Source: CAD feature listing. Evaluate the final solid. Frame: model axes, mm. A direction names the side the tool comes from. Coordinates: 2 decimals unless noted, no trailing zeros. Order: outer loops, then holes, each group sorted by start corner. A loop starts at its lowest first (then second) coordinate and runs counter-clockwise, first axis right, second up.
Autodesk Inventor part; units mm, degrees
ref_plane "YZ Plane" through (0, 0, 0) normal (1, 0, 0) x (0, 1, 0)
ref_plane "XZ Plane" through (0, 0, 0) normal (0, 1, 0) x (-1, 0, 0)
ref_plane "XY Plane" through (0, 0, 0) normal (0, 0, 1) x (1, 0, 0)
sketch "Sketch1" plane through (0, 0, 0) normal (0, 0, 1) x (1, 0, 0)
  line L0 (-16.8009, 21.2415) -> (21.2415, -16.8009)
  line L1 (21.2415, -16.8009) -> (16.8009, -21.2415)
  line L2 (16.8009, -21.2415) -> (-21.2415, 16.8009)
  line L3 (-21.2415, 16.8009) -> (-16.8009, 21.2415)
  line L4 (-16.8009, 21.2415) -> (16.8009, -21.2415) construction
  line L5 (21.2415, -16.8009) -> (-21.2415, 16.8009) construction
  line L6 (-16.8009, 21.2415) -> (36.9991, 21.2415) construction
  line L7 (-21.2415, 16.8009) -> (-24, 16.8009)
  line L8 (16.8009, -21.2415) -> (16.8009, -24)
  line L9 (16.8009, -24) -> (-24, 16.8009)
  line L10 (-16.8009, 21.2415) -> (-16.8009, 24)
  line L11 (21.2415, -16.8009) -> (24, -16.8009)
  line L12 (24, -16.8009) -> (-16.8009, 24)
  line L13 (-24, 16.8009) -> (-24, 12.6863)
  line L14 (16.8009, -24) -> (12.6863, -24)
  line L15 (-24, 12.6863) -> (12.6863, -24)
  line L16 (-24, 16.8009) -> (-11.8721, 28.9288) construction
  line L17 (-24, 16.8009) -> (-6.8486, 16.8009) construction
  point P0 (0, 0)
  dimension "d0" = 53.8
  dimension "d1" = 45
  dimension "d2" = 6.28
  dimension "d5" = 8
  dimension "d72" = 24
  dimension "d73" = 45
extrude "Extrusion1" add sketch "Sketch1" along normal blind 30
ref_plane "Work Plane1" through (16.9, -16.9, -8) normal (-0.7071, -0.7071, 0) x (0, 0, 1)
sketch "Sketch7" plane through (0, 0, 30) normal (0, 0, 1) x (1, 0, 0)
  line L0 (21.2415, -16.8009) -> (24, -16.8009)
  line L1 (24, -16.8009) -> (-16.8009, 24)
  line L2 (-16.8009, 24) -> (-16.8009, 21.2415)
  line L3 (-16.8009, 21.2415) -> (-21.2415, 16.8009)
  line L4 (-21.2415, 16.8009) -> (-24, 16.8009)
  line L5 (-24, 16.8009) -> (-24, 12.6863)
  line L6 (-24, 12.6863) -> (12.6863, -24)
  line L7 (12.6863, -24) -> (16.8009, -24)
  line L8 (16.8009, -24) -> (16.8009, -21.2415)
  line L9 (16.8009, -21.2415) -> (21.2415, -16.8009)
  line L10 (3.5996, 3.5996) -> (-5.6569, -5.6569)
  line L11 (-24, 12.6863) -> (12.6863, -24)
  line L12 (18.1593, -3.761) -> (10.9602, -10.9602)
  line L13 (10.9602, -10.9602) -> (-10.9602, 10.9602)
  line L14 (-10.9602, 10.9602) -> (-3.761, 18.1593)
  line L15 (-3.761, 18.1593) -> (18.1593, -3.761)
  line L16 (18.1593, -3.761) -> (-10.9602, 10.9602) construction
  line L17 (10.9602, -10.9602) -> (-3.761, 18.1593) construction
  line L18 (-10.9602, 10.9602) -> (-10.9602, 18.1593)
  line L19 (24, -16.8009) -> (-16.8009, 24)
  line L20 (10.9602, -10.9602) -> (18.1593, -10.9602)
  point P0 (0, 0)
  dimension "d28" = 31
  dimension "d29" = 0
  dimension "d74" = 0
extrude "Extrusion7" cut sketch "Sketch7" against normal through all contours L20 L12 L1 | L12 L13 L10 L1 | L1 L14 L15 L12 | L10 L13 L14 L1 | L14 L18 L1
sketch "Sketch13" plane through (0, 0, 30) normal (0, 0, 1) x (1, 0, 0)
  line L0 (-10.9602, 18.1593) -> (-16.8009, 24) construction
  line L1 (-16.8009, 24) -> (-16.8009, 21.2415)
  line L2 (-16.8009, 21.2415) -> (-21.2415, 16.8009)
  line L3 (-21.2415, 16.8009) -> (-24, 16.8009)
  line L4 (-24, 16.8009) -> (-24, 12.6863) construction
  line L5 (-24, 12.6863) -> (12.6863, -24) construction
  line L6 (12.6863, -24) -> (16.8009, -24) construction
  line L7 (16.8009, -24) -> (16.8009, -21.2415)
  line L8 (16.8009, -21.2415) -> (21.2415, -16.8009)
  line L9 (21.2415, -16.8009) -> (24, -16.8009)
  line L10 (24.1, -24.6971) -> (24.1, -16.7029) construction
  line L11 (24.1, -16.7029) -> (-16.9409, 24.338) construction
  line L12 (-16.9409, 24.338) -> (-16.9409, 21.2995)
  line L13 (-16.9409, 21.2995) -> (-21.2995, 16.9409)
  line L14 (-21.2995, 16.9409) -> (-24.14, 16.9409)
  line L15 (-24.14, 16.9409) -> (-24.14, 12.6283) construction
  line L16 (-24.14, 12.6283) -> (12.6283, -24.14) construction
  line L17 (12.6283, -24.14) -> (16.9409, -24.14) construction
  line L18 (16.9409, -24.14) -> (16.9409, -21.2995)
  line L19 (16.9409, -21.2995) -> (21.2995, -16.9409)
  line L20 (21.2995, -16.9409) -> (24.2814, -16.9409)
  line L21 (24.2814, -16.9409) -> (53.8994, -46.5588) construction
  line L22 (53.8994, -46.5588) -> (45.9617, -46.5588) construction
  line L23 (45.9617, -46.5588) -> (24.1, -24.6971) construction
  line L24 (16.8009, -24) -> (16.9409, -24)
  line L25 (24, -16.8009) -> (24.1393, -16.9409)
  line L26 (-21.2415, 16.8009) -> (-22.9, 16.8009)
  line L27 (18.1593, -10.9602) -> (10.9602, -10.9602)
  line L28 (10.9602, -10.9602) -> (-10.9602, 10.9602)
  line L29 (-10.9602, 10.9602) -> (-10.9602, 18.1593)
  line L30 (24, -16.8009) -> (18.1593, -10.9602)
  line L31 (-24, 12.6863) -> (-24, 16.8009)
  line L32 (-24, 16.8009) -> (-24, 16.9409)
  line L33 (-16.8009, 24) -> (-16.9409, 24.14)
  point P0 (0, 0)
  point P1 (-22.9, 16.9409)
  dimension "d93" = 0.14
extrude "IM_offset" add sketch "Sketch13" against normal up to surface (30 mm away)
sketch "Skizze14" plane through (12.6863, -24, 30) normal (-0.7071, -0.7071, 0) x (-0.7071, 0.7071, 0)
  line L0 (21.8411, 19.1) -> (30.0411, 19.1)
  line L1 (30.0411, 19.1) -> (30.0411, 10.9)
  line L2 (30.0411, 10.9) -> (21.8411, 10.9)
  line L3 (21.8411, 10.9) -> (21.8411, 19.1)
  line L4 (21.8411, 19.1) -> (30.0411, 10.9) construction
  line L5 (30.0411, 19.1) -> (21.8411, 10.9) construction
  line L6 (0, 30) -> (0, 0) construction
  line L7 (51.8823, 30) -> (51.8823, 0) construction
  line L8 (0, 30) -> (51.8823, 0) construction
  line L9 (51.8823, 0) -> (51.8823, 30) construction
  line L10 (51.8823, 30) -> (0, 0) construction
  line L11 (-2.9094, 0) -> (5.3506, 0) construction
  point P0 (25.9411, 30)
  point P1 (25.9411, 15)
  dimension "d94" = 8.2
  dimension "d95" = 8.2
extrude "Extrusion11" cut sketch "Skizze14" against normal blind 10
sketch "Skizze15" plane through (12.6863, -24, 30) normal (-0.7071, -0.7071, 0) x (-0.7071, 0.7071, 0)
  line L0 (30.0411, 19.1) -> (30.0411, 10.9)
  line L1 (30.0411, 10.9) -> (21.8411, 10.9)
  line L2 (21.8411, 10.9) -> (21.8411, 19.1)
  line L3 (21.8411, 19.1) -> (30.0411, 19.1)
  line L4 (0, 30) -> (51.8823, 30)
  line L5 (0, 30) -> (0, 0)
  line L6 (51.8823, 0) -> (0, 0)
  line L7 (51.8823, 30) -> (51.8823, 0)
  line L8 (51.8823, 30) -> (51.8823, 0)
  line L9 (0, 30) -> (0, 0)
  line L10 (51.8823, 30) -> (0, 0)
  line L11 (0, 0) -> (0, 30)
  line L12 (-2.9094, 30) -> (5.3506, 30)
  line L13 (51.8823, 0) -> (0, 30)
  line L14 (38.4411, 2.5) -> (13.4411, 2.5)
  line L15 (13.4411, 2.5) -> (13.4411, 27.5)
  line L16 (13.4411, 27.5) -> (38.4411, 27.5)
  line L17 (38.4411, 27.5) -> (38.4411, 2.5)
  line L18 (38.4411, 2.5) -> (13.4411, 27.5) construction
  line L19 (13.4411, 2.5) -> (38.4411, 27.5) construction
  point P0 (25.9411, 30)
  point P1 (25.9411, 15)
  dimension "d98" = 25
  dimension "d99" = 25
extrude "Extrusion12" cut sketch "Skizze15" against normal blind 3 contours L3 L2 L13 L15 L16 L17 L10 L0 | L10 L17 L13 L0 | L13 L17 L14 L15 L10 L2 L1 L0 | L2 L10 L15 L13
chamfer "Fase1" distance 2.5 angle 45 4 edges at (3.182, -14.4957, 15) (-5.6569, -5.6569, 27.5) (-14.4957, 3.182, 15) (-5.6569, -5.6569, 2.5)
equation "\"d3\" = MirrorThickness1"
equation "\"MirrorThickness1\" = 30"
properties part number "20_Cube_Insert_Mirror_Holder_wLogo_v3"
1. Ray query, line 1 (X direction, y = 15, z = 23.25); line 2 (Y direction, x = 2.5, z = 28.75). Return the intervals inside material, ascending.
Findings:
line 1: x = -24 to -10.96
line 2: y = -12.05 to -2.5
2. Access query for faces 4 (the face through (23, -16.941, 15)), 5 (the face through (15, -10.96, 15)), 6 (the face through (-14, 4.949, 15)). Directions: +Z, -Z, +X, -X, +Y, -Y. A direction counts if a zero-diameter tool reaches every point of the face in a straight line with its end or side. Return the directions, or none.
Findings:
face 4: +Z, -Z, +X, -Y
face 5: +Z, -Z, +X, +Y
face 6: -X, -Y
3. Draft query along Z for faces 1 (the face through (1.1, -4.7, 15.1)), 2 (the face through (-2, -2, 30)), 3 (the face through (-2, -2, 0)). Return one class per face: released by +Z, released by -Z, zero draft, split by the parting line, or undercut.
Findings:
face 1: undercut
face 2: released by +Z
face 3: released by -Z
4. Section query B-B on z = 20. Return loops of the section in (x, y).
Findings:
outline: (-24, 12.69) - (-16.26, 4.95) - (-12.73, 4.95) - (-12.37, 5.3) - (5.3, -12.37) - (4.95, -12.73) - (4.95, -16.26) - (12.69, -24) - (16.94, -24) - (16.94, -21.3) - (21.3, -16.94) - (24.14, -16.94) - (24, -16.8) - (18.16, -10.96) - (10.96, -10.96) - (-10.96, 10.96) - (-10.96, 18.16) - (-16.94, 24.14) - (-16.94, 21.3) - (-21.3, 16.94) - (-24, 16.94) - close
5. Pin query (flat end, axial travel): P1, Ø6, axis at x = 16, z = 19.5, coming from the +Y side; P2, Ø1.4, axis at y = -22.5, z = 11.5, coming from the +X side; P3, Ø10.5, axis at x = 0, y = -0.5, coming from the -Z side; P4, Ø1.5, axis at y = -11, z = 10.5, coming from the -X side. Return the tip coordinate at first contact, or that it passes through.
Findings:
P1: stops at y = -10.96
P2: stops at x = 16.94
P3: stops at z = 0
P4: stops at x = 3.18
